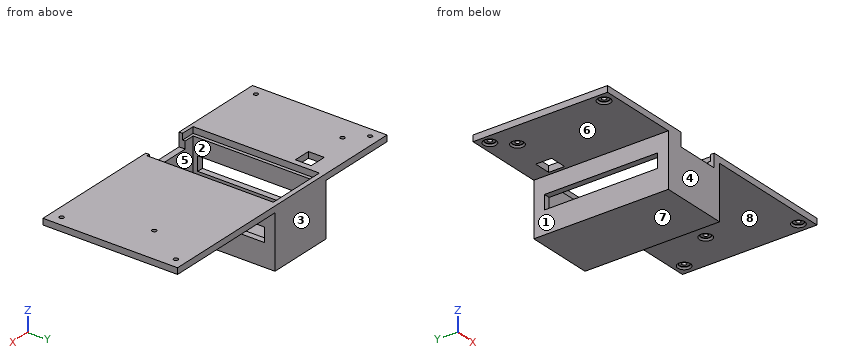
```python
from build123d import *

# Parameters (mm, degrees)
SKETCH1_W                                   = 114.20462943
SKETCH1_H                                   = 55.88
BOSS_EXTRUDE1_DEPTH                         = 2.54
CUT_EXTRUDE2_REACH                          = 4.54
SKETCH2_W                                   = 7.112
SKETCH2_H                                   = 6.604
SKETCH5_W                                   = 27.94
SKETCH5_H                                   = 55.88
BOSS_EXTRUDE2_DEPTH                         = 19.558
SHELL2_T                                    = -2.54
SKETCH6_W                                   = 25.09706722
SKETCH6_H                                   = 52.434836366
CUT_EXTRUDE3_DEPTH                          = 3.54
SKETCH7_W                                   = 5.85197615
SKETCH7_H                                   = 46.976533267
CUT_EXTRUDE4_DEPTH                          = 62.079438962
SKETCH8_W                                   = 18.161
SKETCH8_H                                   = 5.588
CUT_EXTRUDE5_DEPTH                          = 19.558
CBORE_FOR_0_BINDING_HEAD_MACHINE_SC_2_COUNT = 2
CBORE_FOR_0_BINDING_HEAD_MACHINE_SC_2_PITCH = 88.953731343
CBORE_FOR_0_BINDING_HEAD_MACHINE_SC_3_COUNT = 2
CBORE_FOR_0_BINDING_HEAD_MACHINE_SC_3_PITCH = 47.42542097
CBORE_FOR_0_BINDING_HEAD_MACHINE_SC_4_COUNT = 2
CBORE_FOR_0_BINDING_HEAD_MACHINE_SC_4_PITCH = 136.214285903
CBORE_FOR_0_BINDING_HEAD_MACHINE_SC_5_COUNT = 2
CBORE_FOR_0_BINDING_HEAD_MACHINE_SC_5_PITCH = 116.073664451
CBORE_FOR_0_BINDING_HEAD_MACHINE_SC_6_COUNT = 2
CBORE_FOR_0_BINDING_HEAD_MACHINE_SC_6_PITCH = 105.943027259
SKETCH16_W                                  = 27.94
SKETCH16_H                                  = 55.88
BOSS_EXTRUDE3_DEPTH                         = 2.54


with BuildPart() as part:
    # Sketch1 → Boss-Extrude1 (new body)
    with BuildSketch(Plane.XY):
        with Locations((3000.394884782, 13522.309097574)):
            Rectangle(SKETCH1_W, SKETCH1_H)
    extrude(amount=-BOSS_EXTRUDE1_DEPTH)

    # Sketch2 → Cut-Extrude2 (cut, up to next)
    with BuildSketch(Plane(origin=(0, 0, -2.54), x_dir=(-1, 0, 0), z_dir=(0, 0, -1)), mode=Mode.PRIVATE) as cut_extrude2_sk1:
        with Locations((-2971.586819557, 13539.747648461)):
            Rectangle(SKETCH2_W, SKETCH2_H)
    cut_extrude2_tool1 = extrude(cut_extrude2_sk1.sketch, amount=-CUT_EXTRUDE2_REACH, mode=Mode.PRIVATE) & part.part
    add(cut_extrude2_tool1.solids().sort_by_distance((2971.58682, 13539.747648, -2.54))[0], mode=Mode.SUBTRACT)

    # Sketch5 → Boss-Extrude2 (add)
    with BuildSketch(Plane(origin=(0, 0, -2.54), x_dir=(-1, 0, 0), z_dir=(0, 0, -1))):
        with Locations((-2990.402009029, 13522.309097574)):
            Rectangle(SKETCH5_W, SKETCH5_H)
    extrude(amount=BOSS_EXTRUDE2_DEPTH)

    # Shell2
    shell2_openings = [part.faces().sort_by_distance(p)[0] for p in [
        (2990.402009029, 13522.309097574, -22.098),
    ]]
    offset(amount=SHELL2_T, openings=shell2_openings, kind=Kind.INTERSECTION)

    # Sketch6 → Cut-Extrude3 (cut, through all)
    with BuildSketch(Plane(origin=(0, 0, -2.54), x_dir=(-1, 0, 0), z_dir=(0, 0, -1))):
        with Locations((-2990.095388415, 13522.03687782)):
            Rectangle(SKETCH6_W, SKETCH6_H)
    extrude(amount=-CUT_EXTRUDE3_DEPTH, mode=Mode.SUBTRACT)

    # Sketch7 → Cut-Extrude4 (cut, through all)
    with BuildSketch(Plane(origin=(3004.372009029, 0, 0), x_dir=(0, 0, -1), z_dir=(1, 0, 0))):
        with Locations((12.319, 13522.309097574)):
            Rectangle(SKETCH7_W, SKETCH7_H)
    extrude(amount=-CUT_EXTRUDE4_DEPTH, mode=Mode.SUBTRACT)

    # Sketch8 → Cut-Extrude5 (cut)
    with BuildSketch(Plane.XZ.offset(-13494.369097574)):
        with Locations((2992.380051535, -2.794)):
            Rectangle(SKETCH8_W, SKETCH8_H)
    extrude(amount=-CUT_EXTRUDE5_DEPTH, mode=Mode.SUBTRACT)

    # Sketch9 → CBORE for _0 Binding Head Machine Screw1 (revolve, cut)
    with BuildSketch(Plane(origin=(3041.896978852, 13528.711016341, -2.54), x_dir=(0, 1, 0), z_dir=(1, 0, 0))):
        Polygon((0, 0), (0, 2.54), (0.889, 2.54), (0.889, 0.8128), (1.98501, 0.8128), (1.98501, 0.635), (2.62001, 0), align=None)
    cbore_for_0_binding_head_machine_screw1 = revolve(axis=Axis((3041.896978852, 13528.711016341, -8.89), (0, 0, 1)), mode=Mode.SUBTRACT)

    # CBORE for _0 Binding Head Machine Sc 2: CBORE for _0 Binding Head Machine Screw1 ×2
    with Locations(*[Vector(-0.99241101, 0.122964985, 0) * (i * CBORE_FOR_0_BINDING_HEAD_MACHINE_SC_2_PITCH) for i in range(1, CBORE_FOR_0_BINDING_HEAD_MACHINE_SC_2_COUNT)]):
        add(cbore_for_0_binding_head_machine_screw1, mode=Mode.SUBTRACT)

    # Sketch14 → CBORE for _0 Binding Head Machine Screw2 (revolve, cut)
    with BuildSketch(Plane(origin=(3053.204515133, 13546.256494849, -2.54), x_dir=(0, 1, 0), z_dir=(1, 0, 0))):
        Polygon((0, 0), (0, 2.54), (0.889, 2.54), (0.889, 0.8128), (1.98501, 0.8128), (1.98501, 0.635), (2.62001, 0), align=None)
    cbore_for_0_binding_head_machine_screw2 = revolve(axis=Axis((3053.204515133, 13546.256494849, -8.89), (0, 0, 1)), mode=Mode.SUBTRACT)

    # CBORE for _0 Binding Head Machine Sc 3: CBORE for _0 Binding Head Machine Screw2 ×2
    with Locations(*[(0, -i * CBORE_FOR_0_BINDING_HEAD_MACHINE_SC_3_PITCH, 0) for i in range(1, CBORE_FOR_0_BINDING_HEAD_MACHINE_SC_3_COUNT)]):
        add(cbore_for_0_binding_head_machine_screw2, mode=Mode.SUBTRACT)

    # CBORE for _0 Binding Head Machine Sc 4: CBORE for _0 Binding Head Machine Screw2 ×2
    with Locations(*[Vector(-0.937315117, -0.348482957, 0) * (i * CBORE_FOR_0_BINDING_HEAD_MACHINE_SC_4_PITCH) for i in range(1, CBORE_FOR_0_BINDING_HEAD_MACHINE_SC_4_COUNT)]):
        add(cbore_for_0_binding_head_machine_screw2, mode=Mode.SUBTRACT)

    # CBORE for _0 Binding Head Machine Sc 5: CBORE for _0 Binding Head Machine Screw2 ×2
    with Locations(*[Vector(-0.912722345, -0.408580372, 0) * (i * CBORE_FOR_0_BINDING_HEAD_MACHINE_SC_5_PITCH) for i in range(1, CBORE_FOR_0_BINDING_HEAD_MACHINE_SC_5_COUNT)]):
        add(cbore_for_0_binding_head_machine_screw2, mode=Mode.SUBTRACT)

    # CBORE for _0 Binding Head Machine Sc 6: CBORE for _0 Binding Head Machine Screw2 ×2
    with Locations(*[(-i * CBORE_FOR_0_BINDING_HEAD_MACHINE_SC_6_PITCH, 0, 0) for i in range(1, CBORE_FOR_0_BINDING_HEAD_MACHINE_SC_6_COUNT)]):
        add(cbore_for_0_binding_head_machine_screw2, mode=Mode.SUBTRACT)

    # Sketch16 → Boss-Extrude3 (add)
    with BuildSketch(Plane(origin=(0, 0, -22.098), x_dir=(-1, 0, 0), z_dir=(0, 0, -1))):
        with Locations((-2990.402009029, 13522.309097574)):
            Rectangle(SKETCH16_W, SKETCH16_H)
    extrude(amount=BOSS_EXTRUDE3_DEPTH)


solid = part.part
```
Can you work these out from the model? Positions are in its coordinate system, mm. Face numbers are marked on the shaded views. A direction names the side the tool comes from. Give positions to 0.01 mm unless a question says otherwise; leave off trailing zeros. Write each loop counter-clockwise with the first axis right and the second up, starting at its lowest first coordinate (ties: lowest second). Pieces come first, ordered by that corner, then holes. Notation, with made-up numbers: (81, 75) -> (105, 75) arc R16 ccw to (105, 101) -> close; hole circle Ø8 at (-26, 84.5). An arc over 180 degrees is marked (long way). Write item = value, one per line.
(1) Suppose I cut it at D-D on z = -12.75. Write out the boundary of the cut face in (x, y).
Worked out:
outline = (2976.43, 13494.37) -> (3004.37, 13494.37) -> (3004.37, 13498.82) -> (3001.83, 13498.82) -> (3001.83, 13496.91) -> (2978.97, 13496.91) -> (2978.97, 13498.82) -> (2976.43, 13498.82) -> close; (2976.43, 13545.8) -> (2978.97, 13545.8) -> (2978.97, 13547.71) -> (3001.83, 13547.71) -> (3001.83, 13545.8) -> (3004.37, 13545.8) -> (3004.37, 13550.25) -> (2976.43, 13550.25) -> close
(2) I need wall thicknesses on probe 1 along X at (y, z) = (13527, -7.5); probe 2 along Y at (x, z) = (2997, -20.25); probe 3 along X at (y, z) = (13521.5, -1.5). Which ranges of each line are inside material? Lowest first, please. Write a range as from..to.
Worked out:
probe_1 = 2976.43..2978.97, 3001.83..3004.37
probe_2 = 13494.37..13496.91, 13547.71..13550.25
probe_3 = 2943.29..2977.55, 3002.64..3057.5
(3) Thinking about a two-plate mould opening in Y: for the marked faces 1, 2, 3 and 4, which applies, released by +Y, released by -Y, zero draft, split by the parting line, or undercut?
Worked out:
face_1 = zero draft
face_2 = undercut
face_3 = released by +Y
face_4 = released by -Y
(4) Suppose I cut it at A-A on z = -8. Write out the boundary of the cut face in (x, y), then the cut area to 3 significant figures.
Worked out:
outline = (2976.43, 13494.37) -> (3004.37, 13494.37) -> (3004.37, 13550.25) -> (2976.43, 13550.25) -> close; hole (2978.97, 13496.91) -> (3001.83, 13496.91) -> (3001.83, 13547.71) -> (2978.97, 13547.71) -> close
area = 400 mm^2
(5) Suppose I cut it at B-B on y = 13504. Write out the boundary of the cut face in (x, z).
Worked out:
outline = (2943.29, -2.54) -> (2976.43, -2.54) -> (2976.43, -9.39) -> (2978.97, -9.39) -> (2978.97, -2.54) -> (2977.55, -2.54) -> (2977.55, 0) -> (2943.29, 0) -> close; (2976.43, -24.64) -> (3004.37, -24.64) -> (3004.37, -15.24) -> (3001.83, -15.24) -> (3001.83, -22.1) -> (2978.97, -22.1) -> (2978.97, -15.24) -> (2976.43, -15.24) -> close; (3001.83, -9.39) -> (3004.37, -9.39) -> (3004.37, -2.54) -> (3057.5, -2.54) -> (3057.5, 0) -> (3002.64, 0) -> (3002.64, -2.54) -> (3001.83, -2.54) -> close
(6) I'm going to push flat-ended pins straight in: P1, Ø1.5, axis at y = 13544.5, z = -12, coming from the +X side (1 decimal); P2, Ø1.2, axis at x = 2947, y = 13499.5, coming from the -Z side; P3, Ø12, axis at y = 13516, z = -12.5, coming from the +X side; P4, Ø3, axis at x = 3053, y = 13498, coming from the -Z side. Where does each tip first touch, or does it pass through?
Worked out:
P1 = through
P2 = -1.73
P3 = 3004.37
P4 = -2.28
(7) Suppose I cut it at C-C on x = 2992. Write out the boundary of the cut face in (y, z), then the cut area to 3 significant figures.
Worked out:
outline = (13494.37, -24.64) -> (13550.25, -24.64) -> (13550.25, 0) -> (13548.25, 0) -> (13548.25, -2.54) -> (13547.71, -2.54) -> (13547.71, -22.1) -> (13496.91, -22.1) -> (13496.91, -5.59) -> (13494.37, -5.59) -> close
area = 239 mm^2
(8) For the marked faces 5, 6, 7 and 8, which set-ups out of +Z, -Z, +X, -X, +Y, -Y let a thin tool reach every point of the face, with its end or its side?
Worked out:
face_5 = +Z
face_6 = -Z, -X, +Y, -Y
face_7 = -Z, +X, -X, +Y, -Y
face_8 = -Z, +X, +Y, -Y
